Build history of the part. All positions in model axes, mm. Face numbers are marked on the shaded views. Coordinates: 2 decimals unless noted, no trailing zeros. Use a Markdown table: item, result. Add a question column.
Autodesk Inventor part; units mm, degrees
ref_plane "YZ Plane" through (0, 0, 0) normal (1, 0, 0) x (0, 1, 0)
ref_plane "XZ Plane" through (0, 0, 0) normal (0, 1, 0) x (-1, 0, 0)
ref_plane "XY Plane" through (0, 0, 0) normal (0, 0, 1) x (1, 0, 0)
sketch "Эскиз1" plane through (0, 0, 0) normal (0, 1, 0) x (-1, 0, 0)
  circle A0 centre (0, 0) radius 20
  ellipse E0 centre (0, 0) end of major axis (0, -55) minor radius 40 (40, 0) -> (0, 55) ccw
  ellipse E1 centre (0, 0) end of major axis (0, -55) minor radius 40 (-40, 0) -> (0, -55) ccw
  arc A1 (0, -40) -> (40, 0) centre (0, 0) ccw
  arc A2 (0, 40) -> (-40, 0) centre (0, 0) ccw
  line L0 (0, 55) -> (0, 40)
  line L1 (0, -40) -> (0, -55)
  line L2 (0, -40) -> (0, -55)
  line L3 (0, 40) -> (0, 55)
  dimension "d0" = 40
  dimension "d2" = 55
  dimension "d3" = 55
extrude "Выдавливание1" add sketch "Эскиз1" along normal blind 350
sketch "Эскиз2" plane through (0, 350, 0) normal (0, 1, 0) x (1, 0, 0)
  point P0 (0, 0)
hole "Отверстие1" at (0, 350, 0) direction (0, -1, 0) diameter 60 depth 15
sketch "Эскиз3" plane through (0, 350, 0) normal (0, 1, 0) x (1, 0, 0)
  line L0 (0, 0) -> (-20, 0)
  circle A0 centre (0, 0) radius 20
  line L1 (0, 0) -> (0, 20)
  line L2 (0, 0) -> (0, -20)
  line L3 (0, 0) -> (20, 0)
hole "Отверстие2" at (-20, 350, 0) at (0, 350, -20) at (20, 350, 0) at (0, 350, 20) direction (0, -1, 0) diameter 10 depth 45
sketch "Эскиз4" plane through (0, 0, 0) normal (0, -1, 0) x (1, 0, 0)
  circle A0 centre (0, 0) radius 30
hole "Отверстие3" at (0, 0, 0) direction (0, 1, 0) diameter 60 depth 15
sketch "Эскиз5" plane through (0, 0, 0) normal (0, -1, 0) x (1, 0, 0)
  line L0 (0, 0) -> (-14.1421, -14.1421)
  line L1 (0, 0) -> (20, 0) construction
  line L2 (0, 0) -> (-14.1421, 14.1421)
  arc A0 (-4.9608, 19.375) -> (-19.375, 4.9608) centre (0, 0) ccw
  line L3 (0, 0) -> (14.1421, 14.1421)
  line L4 (0, 0) -> (14.1421, -14.1421)
  dimension "d27" = 20
  dimension "d28" = 135
hole "Отверстие4" at (14.1421, 0, -14.1421) at (-14.1421, 0, 14.1421) at (14.1421, 0, 14.1421) at (-14.1421, 0, -14.1421) direction (0, 1, 0) diameter 10 depth 45
sketch "Эскиз6" plane through (0, 0, 0) normal (0, -1, 0) x (1, 0, 0)
  line L0 (0, 0) -> (0, 25)
  arc A0 (4.9608, 19.375) -> (-4.9608, 19.375) centre (0, 20) ccw
  line L1 (0, 0) -> (-25, 0)
  arc A1 (-19.375, 4.9608) -> (-19.375, -4.9608) centre (-20, 0) ccw
  line L2 (0, 0) -> (0, -25)
  arc A2 (-4.9608, -19.375) -> (4.9608, -19.375) centre (0, -20) ccw
  line L3 (0, 0) -> (25, 0)
  arc A3 (19.375, -4.9608) -> (19.375, 4.9608) centre (20, 0) ccw
hole "Отверстие5" at (0, 0, -25) at (-25, 0, 0) at (0, 0, 25) at (25, 0, 0) direction (0, 1, 0) diameter 6 depth 25
sketch "Эскиз7" plane through (0, 350, 0) normal (0, 1, 0) x (1, 0, 0)
  line L0 (0, 0) -> (-17.6771, 17.6782)
  arc A0 (-10.1924, 17.208) -> (-17.208, 10.1924) centre (-14.1421, 14.1421) ccw
  line L1 (0, 0) -> (-17.6782, -17.6771)
  arc A1 (-17.208, -10.1924) -> (-10.1924, -17.208) centre (-14.1421, -14.1421) ccw
  line L2 (0, 0) -> (17.6771, -17.6782)
  arc A2 (10.1924, -17.208) -> (17.208, -10.1924) centre (14.1421, -14.1421) ccw
  line L3 (0, 0) -> (17.6782, 17.6771)
  arc A3 (17.208, 10.1924) -> (10.1924, 17.208) centre (14.1421, 14.1421) ccw
hole "Отверстие6" at (-17.6782, 350, 17.6771) at (-17.6771, 350, -17.6782) at (17.6782, 350, -17.6771) at (17.6771, 350, 17.6782) direction (0, -1, 0) diameter 6 depth 25
properties part number "Барабан" material "Сталь, литейная"
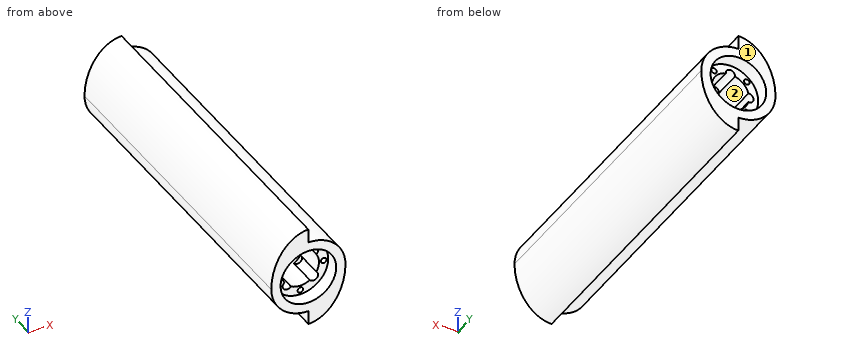
(1) Drop flat-ended pins along their axis: P1, Ø6.5, axis at x = -17, z = 18, coming from the +Y side; P2, Ø4, axis at x = 15, y = 60.5, coming from the +Z side; P3, Ø1, axis at x = 1.5, y = 167, coming from the +Z side; P4, Ø4, axis at x = 1, y = 145.5, coming from the +Z side. Give the stop position or say it passes through.
(2) Mould opens along X. For the marked faces 1 and 2 say: released by +X, released by -X, zero draft, split by the parting line, or undercut.
(3) Drill centre lines: line 1 along X through (y, z) = (9, 0); line 2 along X through (y, z) = (304, -4); line 3 along Z through (x, y) = (-5, 160). Where is each one in solid material? Low to high. Write a range as from..to.
Solutions:
| question | item | result |
|---|---|---|
| 1 | P1 | y = 335 |
| 1 | P2 | z = 37.83 |
| 1 | P3 | z = 39.99 |
| 1 | P4 | z = 55 |
| 2 | face 1 | zero draft |
| 2 | face 2 | undercut |
| 3 | line 1 | -40..-30, 30..40 |
| 3 | line 2 | -39.8..-19.6, 19.6..39.89 |
| 3 | line 3 | -39.69..-19.36, 19.36..54.57 |
